Design review of the part built by this model. Coordinates are the model's own, in mm. Face numbers are marked on the shaded views. A direction names the side the tool comes from. Round coordinates to 2 decimals unless told otherwise and drop trailing zeros. Order: outer loops, then holes, each group sorted by start corner. A loop starts at its lowest first (then second) coordinate and runs counter-clockwise, first axis right, second up.
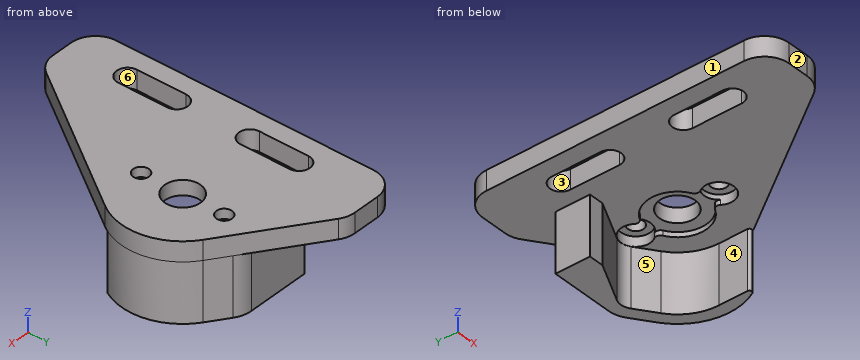
from build123d import *

# Parameters (mm, degrees)
SKETCH1_R           = 3.65
SKETCH1_R_2         = 1.6
BOSS_EXTRUDE1_DEPTH = 2
SKETCH2_R           = 3
CUT_EXTRUDE1_DEPTH  = 2
SKETCH3_R           = 6
CUT_EXTRUDE2_DEPTH  = 1
FILLET1_R           = 1
BOSS_EXTRUDE2_DEPTH = 12


with BuildPart() as part:
    # Sketch1 → Boss-Extrude1 (new, symmetric)
    with BuildSketch(Plane.XY):
        with BuildLine():
            Line((-24, 18.662172818), (-24, -33.930861026))
            ThreePointArc((-24, -33.930861026), (-22.535533906, -37.466394932), (-19, -38.930861026))
            Line((-19, -38.930861026), (-14.602835253, -38.930861026))
            ThreePointArc((-14.602835253, -38.930861026), (-12.294092187, -38.365915192), (-10.507075031, -36.798743208))
            Line((-10.507075031, -36.798743208), (10.239400554, -7.169705454))
            ThreePointArc((10.239400554, -7.169705454), (12.310096913, 2.170602221), (7.169705454, 10.239400554))
            Line((7.169705454, 10.239400554), (-10.708611763, 22.757933039))
            ThreePointArc((-10.708611763, 22.757933039), (-12.072964947, 23.430757572), (-13.576493944, 23.662172818))
            Line((-13.576493944, 23.662172818), (-19, 23.662172818))
            ThreePointArc((-19, 23.662172818), (-22.535533906, 22.197706724), (-24, 18.662172818))
        make_face()
        Circle(SKETCH1_R, mode=Mode.SUBTRACT)
        with Locations((0, 8.5)):
            Circle(SKETCH1_R_2, mode=Mode.SUBTRACT)
        with Locations((0, -8.5)):
            Circle(SKETCH1_R_2, mode=Mode.SUBTRACT)
        with BuildLine():
            Line((-15.75, 8.5), (-15.75, -1.5))
            ThreePointArc((-15.75, -1.5), (-18, -3.75), (-20.25, -1.5))
            Line((-20.25, -1.5), (-20.25, 8.5))
            ThreePointArc((-20.25, 8.5), (-18, 10.75), (-15.75, 8.5))
        make_face(mode=Mode.SUBTRACT)
        with BuildLine():
            Line((-15.75, -16.5), (-15.75, -26.5))
            ThreePointArc((-15.75, -26.5), (-18, -28.75), (-20.25, -26.5))
            Line((-20.25, -26.5), (-20.25, -16.5))
            ThreePointArc((-20.25, -16.5), (-18, -14.25), (-15.75, -16.5))
        make_face(mode=Mode.SUBTRACT)
    extrude(amount=BOSS_EXTRUDE1_DEPTH, both=True)

    # Sketch2 → Cut-Extrude1 (cut)
    with BuildSketch(Plane(origin=(0, 0, -2), x_dir=(-1, 0, 0), z_dir=(0, 0, -1))):
        with Locations((0, 8.5)):
            Circle(SKETCH2_R)
        with Locations((0, -8.5)):
            Circle(SKETCH2_R)
    extrude(amount=-CUT_EXTRUDE1_DEPTH, mode=Mode.SUBTRACT)

    # Sketch3 → Cut-Extrude2 (cut)
    with BuildSketch(Plane(origin=(0, 0, -2), x_dir=(-1, 0, 0), z_dir=(0, 0, -1))):
        Circle(SKETCH3_R)
    extrude(amount=-CUT_EXTRUDE2_DEPTH, mode=Mode.SUBTRACT)

    # Fillet1
    fillet1_edges = [part.edges().sort_by_distance(p)[0] for p in [
        (-1.383838376, -5.838235294, -1.5),
        (1.383838376, -5.838235294, -1.5),
        (-1.383838376, 5.838235294, -1.5),
        (1.383838376, 5.838235294, -1.5),
    ]]
    fillet(fillet1_edges, radius=FILLET1_R)

    # Sketch4 → Boss-Extrude2 (add)
    with BuildSketch(Plane(origin=(0, 0, -2), x_dir=(-1, 0, 0), z_dir=(0, 0, -1))):
        with BuildLine():
            Line((9.8, 7), (1.357173626, 11.217114259))
            ThreePointArc((1.357173626, 11.217114259), (-0.22398046, 11.528937586), (-1.742070725, 10.987934834))
            Line((-1.742070725, 10.987934834), (-5.735764364, 8.191520443))
            ThreePointArc((-5.735764364, 8.191520443), (-8.870108332, 4.617486132), (-10, 0))
            Line((-10, 0), (-10, -5.809475019))
            ThreePointArc((-10, -5.809475019), (-10.375, -6.293597938), (-10.9375, -6.051536478))
            ThreePointArc((-10.9375, -6.051536478), (-12.178521244, 2.8166683), (-7.169705454, 10.239400554))
            Line((-7.169705454, 10.239400554), (-3.176011816, 13.035814944))
            ThreePointArc((-3.176011816, 13.035814944), (-1.665070445, 13.78092877), (0, 14.037207624))
            Line((0, 14.037207624), (12.8, 14.037207624))
            Line((12.8, 14.037207624), (12.8, 7))
            Line((12.8, 7), (9.8, 7))
        make_face()
    extrude(amount=BOSS_EXTRUDE2_DEPTH)


solid = part.part
1) Take a section at C-C on x = -8.5. Give the boundary of the cut face in (y, z), plus the area to 3 significant figures.
Results:
outline: (-33.93, -2) - (7.65, -2) - (7.65, -14) - (14.04, -14) - (14.04, -2) - (21.21, -2) - (21.21, 2) - (-33.93, 2) - close
area: 297 mm2
2) Take a section at D-D on y = -29.5. Give the boundary of the cut face in (x, z).
Results:
outline: (-24, -2) - (-5.4, -2) - (-5.4, 2) - (-24, 2) - close
3) Take a section at B-B on x = -17.5. Give the boundary of the cut face in (y, z).
Results:
outline: (-38.93, -2) - (-28.69, -2) - (-28.69, 2) - (-38.93, 2) - close; (-14.31, -2) - (-3.69, -2) - (-3.69, 2) - (-14.31, 2) - close; (10.69, -2) - (23.66, -2) - (23.66, 2) - (10.69, 2) - close
4) Clearance check with flat-ended pins moving along their axes: P1, Ø1.8, axis at x = 1, y = 7.5, coming from the -Z side; P2, Ø8, axis at y = 9, z = -10.5, coming from the -X side; P3, Ø3, axis at x = 0, y = -8.5, coming from the -Z side; P4, Ø1.5, axis at x = -20, y = -32.5, coming from the -Z side. State where each tip first meets the part, or that it passes through.
Results:
P1: stops at z = 0
P2: stops at x = -12.8
P3: passes through
P4: stops at z = -2
5) For the marked faces 4, 5 and 6, list the 3-axis set-ups (+Z, -Z, +X, -X, +Y, -Y) from which the entire face can be reached by the end or side of a thin tool; tool diameter is ignored.
Results:
face 4: -Z, -X, -Y
face 5: -Z, -Y
face 6: +Z, -Z
6) The part is to be moulded in two halves that separate along Y. For the marked faces 1, 2 and 3, say which applies: released by +Y, released by -Y, zero draft, split by the parting line, or undercut.
Results:
face 1: zero draft
face 2: released by -Y
face 3: undercut
7) To check wall thickness, follow line 1 along X through (y, z) = (0, 0.85); line 2 along Y through (x, z) = (0, 0.8); line 3 along X through (y, z) = (8.5, -1.3). State the ranges of each line that lie inside material, in increasing order.
Results:
line 1: x = -24 to -20.25, -15.75 to -3.65, 3.65 to 12.5
line 2: y = -21.79 to -10.1, -6.9 to -3.65, 3.65 to 6.9, 10.1 to 15.26
line 3: x = -24 to -20.25, -15.75 to -3, 3 to 9.17
8) Take a section at A-A on z = -6.25. Give the boundary of the cut face in (x, y).
Results:
outline: (-12.8, 7) - (-9.8, 7) - (-1.36, 11.22) arc R3.04 cw to (1.74, 10.99) - (5.74, 8.19) arc R10 cw to (10, 0) - (10, -5.81) arc R0.5 ccw to (10.94, -6.05) arc R12.5 ccw to (7.17, 10.24) - (3.18, 13.04) arc R5.54 ccw to (0, 14.04) - (-12.8, 14.04) - close
